Could you check a few things on this drawing? It's one solid part, dimensions in mm from its lowest x, y, z. A direction names the side the tool comes from. Give positions to 0.01 mm unless a question says otherwise; leave off trailing zeros. Order: outer loops, then holes, each group sorted by start corner. A loop starts at its lowest first (then second) coordinate and runs counter-clockwise, first axis right, second up. Notation, with made-up numbers: M 45,79 L 67,79 A22 ccw 67,97 Z; hole C 72,29 d8. An arc over 180 degrees is marked long. Use one line per item in the form item = value. Start each with the question number.
1. I want a section at B-B, the plane z = 35. List the corners of the cut face in (x, y) for me, and give its area (3 significant figures).
2. Will these pins go through, and if not, where does the flat tip stop? P1, Ø2, axis at x = 13, y = 2.5, coming from the +Z side; P2, Ø1, axis at x = 19, z = 26.5, coming from the +Y side; P3, Ø9, axis at x = 6.5, z = 45.5, coming from the +Y side; P4, Ø25, axis at x = 38, y = 44, coming from the -Z side.
3. For the marked faces 1, 2, 3, 4 and 5, which set-ups out of +Z, -Z, +X, -X, +Y, -Y let a thin tool reach every point of the face, with its end or its side?
4. I want a section at C-C, the plane y = 26.5. List the corners of the cut face in (x, z) for me.
5. I want a section at D-D, the plane y = 41. List the corners of the cut face in (x, z) for me.
6. I need wall thicknesses on L1, parallel to Y at x = 38, z = 62.25; L2, parallel to Z at x = 46.5, y = 31; L3, parallel to Z at x = 49, y = 27.5. Which ranges of each line are inside material? Lowest first, please.
7. I want a section at A-A, the plane x = 38. List the corners of the cut face in (y, z) for me.
8. We'd pull the mould along Y, two halves only. Please class the marked faces 6, 7 and 8: +Y half, -Y half, draft (parallel to the pull), parting line (faces both ways), or undercut.
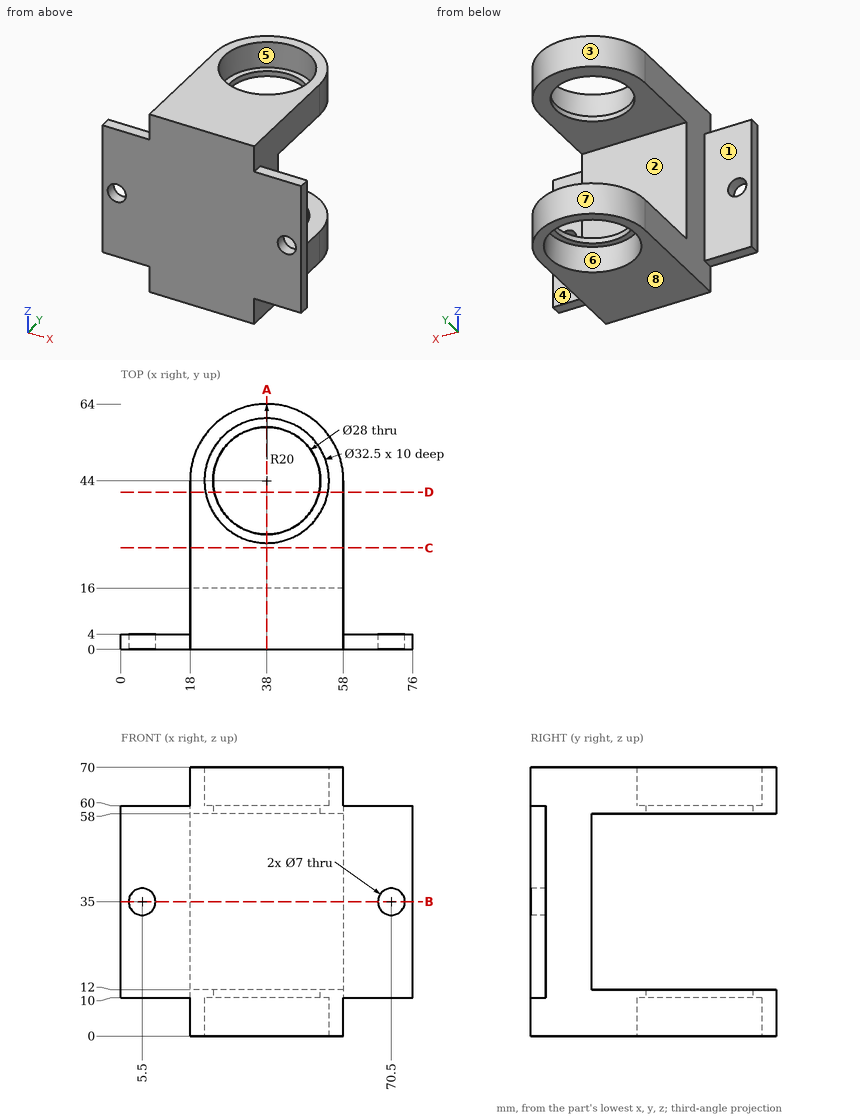
Check result:
q1.outline = M 0,0 L 2,0 L 2,4 L 0,4 Z; M 9,0 L 67,0 L 67,4 L 58,4 L 58,16 L 18,16 L 18,4 L 9,4 Z; M 74,0 L 76,0 L 76,4 L 74,4 Z
q1.area = 728 mm2
q2.P1 = 60
q2.P2 = 16
q2.P3 = 4
q2.P4 = through
q3.face_1 = +Z, -Z, -X, +Y
q3.face_2 = +X, -X, +Y
q3.face_3 = +Z, -Z, +Y
q3.face_4 = +Z, -Z, +X, +Y
q3.face_5 = +Z
q4.outline = M 18,0 L 58,0 L 58,12 L 18,12 Z; M 18,58 L 58,58 L 58,70 L 18,70 Z
q5.outline = M 18,0 L 22.03,0 L 22.03,10 L 24.33,10 L 24.33,12 L 18,12 Z; M 18,58 L 24.33,58 L 24.33,60 L 22.03,60 L 22.03,70 L 18,70 Z; M 51.67,10 L 53.97,10 L 53.97,0 L 58,0 L 58,12 L 51.67,12 Z; M 51.67,58 L 58,58 L 58,70 L 53.97,70 L 53.97,60 L 51.67,60 Z
q6.L1 = 0 to 27.75, 60.25 to 64
q6.L2 = 10 to 12, 58 to 60
q6.L3 = 0 to 12, 58 to 70
q7.outline = M 0,0 L 27.75,0 L 27.75,10 L 30,10 L 30,12 L 16,12 L 16,58 L 30,58 L 30,60 L 27.75,60 L 27.75,70 L 0,70 Z; M 58,10 L 60.25,10 L 60.25,0 L 64,0 L 64,12 L 58,12 Z; M 58,58 L 64,58 L 64,70 L 60.25,70 L 60.25,60 L 58,60 Z
q8.face_6 = undercut
q8.face_7 = +Y half
q8.face_8 = draft
